from build123d import *

# Parameters (mm, degrees)
SKETCH1_R               = 16.5
BOSS_EXTRUDE1_DEPTH     = 20
SKETCH3_R               = 7.5
CUT_EXTRUDE2_DEPTH      = 31.732718721
SKETCH7_R               = 11.5
SKETCH7_R_2             = 7.5
CUT_EXTRUDE3_DEPTH      = 14
CUT_EXTRUDE4_REACH      = 32.733
CUT_EXTRUDE4_END_RADIUS = 11.5
CIRPATTERN1_COUNT       = 3


with BuildPart() as part:
    # Sketch1 → Boss-Extrude1 (new body)
    with BuildSketch(Plane(origin=(0, 0, 0), x_dir=(1, 0, 0), z_dir=(0, 1, 0))):
        with Locations(Location((0, 0, 0), (0, 0, 270))):
            Circle(SKETCH1_R)
    extrude(amount=BOSS_EXTRUDE1_DEPTH)

    # Sketch3 → Cut-Extrude2 (cut, through all)
    with BuildSketch(Plane.XZ):
        with Locations(Location((0, 0, 0), (0, 0, 270))):
            Circle(SKETCH3_R)
    extrude(amount=-CUT_EXTRUDE2_DEPTH, mode=Mode.SUBTRACT)

    # Sketch7 → Cut-Extrude3 (cut)
    with BuildSketch(Plane.XZ):
        with Locations(Location((0, 0, 0), (0, 0, 270))):
            Circle(SKETCH7_R)
        with Locations(Location((0, 0, 0), (0, 0, 270))):
            Circle(SKETCH7_R_2, mode=Mode.SUBTRACT)
    extrude(amount=-CUT_EXTRUDE3_DEPTH, mode=Mode.SUBTRACT)

    # Cut-Extrude4: up to this cylinder (the profile starts inside it)
    cut_extrude4_end = Plane(origin=(2, 5.122343, 0), z_dir=(0, -1, 0)) * Cylinder(CUT_EXTRUDE4_END_RADIUS, 89.466, mode=Mode.PRIVATE)
    # Sketch12 → Cut-Extrude4 (cut, up to the surface)
    with BuildSketch(Plane(origin=(0, 0, 0), x_dir=(0, 0, -1), z_dir=(1, 0, 0)), mode=Mode.PRIVATE) as cut_extrude4_sk1:
        Polygon((-8, -0.446060188), (-8, 8.2), (8, 8.2), (8, 4.1), (-3.5, 4.1), (-3.5, -0.446060188), align=None)
    cut_extrude4_tool1 = extrude(cut_extrude4_sk1.sketch, amount=CUT_EXTRUDE4_REACH, mode=Mode.PRIVATE) & cut_extrude4_end
    cut_extrude4 = cut_extrude4_tool1.solids().sort_by_distance((0, 5.122343, 1.366872))[0]
    add(cut_extrude4, mode=Mode.SUBTRACT)

    # CirPattern1: Cut-Extrude4 ×3 about axis
    cirpattern1_axis = Axis((0, 0, 0), (0, 1, 0))
    for i in range(1, CIRPATTERN1_COUNT):
        add(cut_extrude4.rotate(cirpattern1_axis, i * 360 / CIRPATTERN1_COUNT), mode=Mode.SUBTRACT)


solid = part.part
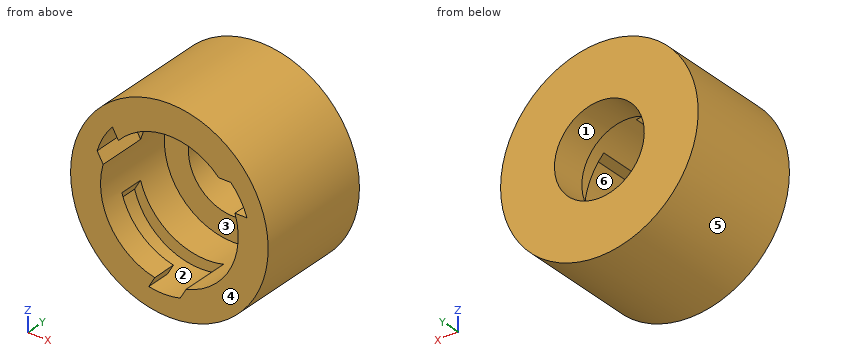
Input: part model. Units: mm. Frame: model coordinates. Face numbers are marked on the shaded views. A direction names the side the tool comes from. Give positions to 0.01 mm unless a question says otherwise; leave off trailing zeros. Loops run counter-clockwise (first coordinate to the right, second up) from the corner with the lowest first, then second, coordinate; pieces in that order, holes last. Notation, with made-up numbers: (-24, -32.5) -> (23, -32.5) arc R34 ccw to (23, 2.5) -> close; hole circle Ø11 at (-37, 78.25). An arc over 180 degrees is marked (long way). Answer as a JSON object with one key per item and string values. Group by question number.
Item 1: Pin query (flat end, axial travel): P1, Ø4, axis at y = 12, z = 3.5, coming from the -X side; P2, Ø6, axis at x = -8.5, y = 17.5, coming from the -Z side; P3, Ø5, axis at x = -5, z = 7, coming from the -Y side. Return the tip coordinate at first contact, or that it passes through.
Item 2: Cut plane C-C, the plane x = -6.5. Return the cut outline in (y, z), and give its area (3 significant figures).
Item 3: Line query: probe 1 along X at (y, z) = (4.75, 0); probe 2 along X at (y, z) = (17.45, 0); probe 3 along Y at (x, z) = (-6.5, 11). Output: solid intervals per line, ascending.
Item 4: Cut plane B-B, the plane y = 5. Return the cut outline in (x, z), and give its area (3 significant figures).
Item 5: Cut plane D-D, the plane z = -7. Return the cut outline in (x, y).
Item 6: Cut plane A-A, the plane z = 0. Return the cut outline in (x, y), and give its area (3 significant figures).
Item 7: Pull-direction query (X, two-part tool) for the marked faces 4, 5 and 6; classes: released by +X, released by -X, zero draft, split by the parting line, or undercut.
Item 8: Reachability of the marked faces 1, 2 and 3 from +Z, -Z, +X, -X, +Y, -Y: full face, straight path, thin tool, end or side. Return the list, or none.
Checks:
{
 "1": {"P1": "stops at x = -16.43", "P2": "stops at z = -15.56", "P3": "stops at y = 14"},
 "2": {"outline": "(0, -15.17) -> (20, -15.17) -> (20, -3.74) -> (14, -3.74) -> (14, -9.49) -> (8.2, -9.49) -> (8.2, -11.83) -> (4.1, -11.83) -> (4.1, -9.49) -> (0, -9.49) -> close; (0, 9.49) -> (4.1, 9.49) -> (4.1, 11.83) -> (8.2, 11.83) -> (8.2, 9.49) -> (14, 9.49) -> (14, 3.74) -> (20, 3.74) -> (20, 15.17) -> (0, 15.17) -> close", "area": "277 mm²"},
 "3": {"probe 1": "x = -16.5 to -11.5, 13.5 to 16.5", "probe 2": "x = -16.5 to -7.5, 7.5 to 16.5", "probe 3": "y = 0 to 4.1, 8.2 to 20"},
 "4": {"outline": "circle Ø33 at (0, 0); hole (-12.06, -4.89) arc R11.5 ccw to (1.8, -12.89) -> (2.8, -11.15) arc R11.5 ccw to (8.26, -8) -> (10.26, -8) arc R11.5 ccw to (10.26, 8) -> (8.26, 8) arc R11.5 ccw to (2.8, 11.15) -> (1.8, 12.89) arc R11.5 ccw to (-12.06, 4.89) -> (-11.06, 3.15) arc R11.5 ccw to (-11.06, -3.15) -> close", "area": "344 mm²"},
 "5": {"outline": "(-14.94, 0) -> (-9.12, 0) -> (-9.12, 4.1) -> (-11.22, 4.1) -> (-11.22, 8.2) -> (-9.12, 8.2) -> (-9.12, 14) -> (-2.69, 14) -> (-2.69, 20) -> (-14.94, 20) -> close; (2.69, 14) -> (9.12, 14) -> (9.12, 8.2) -> (11.12, 8.2) -> (11.12, 4.1) -> (9.12, 4.1) -> (9.12, 0) -> (14.94, 0) -> (14.94, 20) -> (2.69, 20) -> close"},
 "6": {"outline": "(-16.5, 0) -> (-11.5, 0) -> (-11.5, 14) -> (-7.5, 14) -> (-7.5, 20) -> (-16.5, 20) -> close; (7.5, 14) -> (11.5, 14) -> (11.5, 8.2) -> (13.5, 8.2) -> (13.5, 4.1) -> (11.5, 4.1) -> (11.5, 0) -> (16.5, 0) -> (16.5, 20) -> (7.5, 20) -> close", "area": "240 mm²"},
 "7": {"face 4": "zero draft", "face 5": "split by the parting line", "face 6": "undercut"},
 "8": {"face 1": "+Y, -Y", "face 2": "none", "face 3": "-Y"}
}
